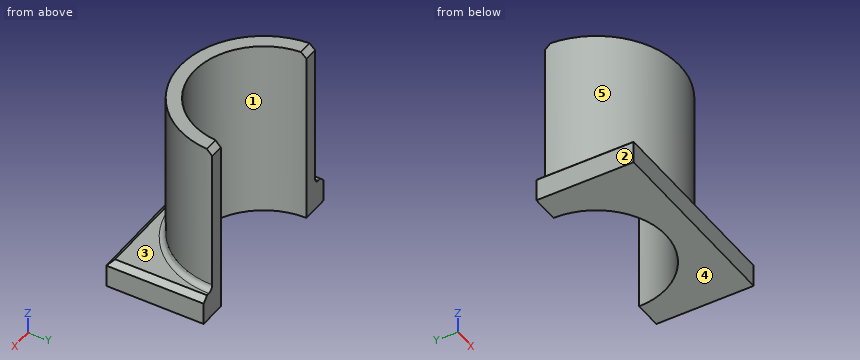
```python
from build123d import *

# Parameters (mm, degrees)
PAD_DEPTH    = 33.02
PAD001_DEPTH = 5.08
FILLET_R     = 1.016
CHAMFER_SIZE = 1


with BuildPart() as part:
    # Sketch001 → Pad (new body)
    with BuildSketch(Plane.XY):
        with BuildLine():
            ThreePointArc((-12.7, 0), (0, -12.7), (12.7, 0))
            Line((12.7, 0), (15.24, 0))
            ThreePointArc((-15.24, 0), (0, -15.24), (15.24, 0))
            Line((-15.24, 0), (-12.7, 0))
        make_face()
    extrude(amount=PAD_DEPTH)

    # Sketch → Pad001 (join)
    with BuildSketch(Plane.XY):
        with BuildLine():
            Line((-17.78, 0), (-17.78, -17.78))
            Line((-17.78, -17.78), (17.78, -17.78))
            Line((17.78, -17.78), (17.78, 0))
            Line((12.7, 0), (17.78, 0))
            ThreePointArc((-12.7, 0), (0, -12.7), (12.7, 0))
            Line((-17.78, 0), (-12.7, 0))
        make_face()
    extrude(amount=PAD001_DEPTH)

    # Fillet
    fillet_edges = [part.edges().sort_by_distance(p)[0] for p in [
        (0, -15.24, 5.08),
    ]]
    fillet(fillet_edges, radius=FILLET_R)

    # Chamfer
    chamfer_edges = [part.edges().sort_by_distance(p)[0] for p in [
        (-13.97, 0, 33.02),
        (13.97, 0, 33.02),
        (-17.78, -8.89, 5.08),
        (17.78, -8.89, 5.08),
        (0, -17.78, 5.08),
    ]]
    chamfer(chamfer_edges, length=CHAMFER_SIZE)


solid = part.part
```
Source: CAD feature listing. Evaluate the final solid. Frame: model axes, mm. Face numbers are marked on the shaded views. A direction names the side the tool comes from. Coordinates: 2 decimals unless noted, no trailing zeros. Order: outer loops, then holes, each group sorted by start corner. A loop starts at its lowest first (then second) coordinate and runs counter-clockwise, first axis right, second up. Notation, with made-up numbers: M 33,5 L 56,5 A18 ccw 56,39 Z; hole C 12,-40 d5. An arc over 180 degrees is marked long. Write each question's results on one line, items separated by ' | '. Start each with the question number.
1) Section query A-A (x = 0). Return the cut outline in (y, z).
2) Line query: line 1 (Z direction, x = -16, y = -9.25); line 2 (X direction, y = -6.75, z = 11); line 3 (X direction, y = -10.75, z = 19.5). Output: solid intervals per line, ascending. Write a range as from..to.
3) Draft query along X for the marked faces 1, 2 and 3. Return one class per face: released by +X, released by -X, zero draft, split by the parting line, or undercut.
4) Access query for the marked faces 4 and 5. Directions: +Z, -Z, +X, -X, +Y, -Y. A direction counts if a zero-diameter tool reaches every point of the face in a straight line with its end or side. Return the directions, or none.
5) Section query B-B (z = 27). Return the cut outline in (x, y), plus the area to 3 significant figures.
6) Contact query for flat-ended pins moving along their axis: pin 1 Ø3 at (y, z) = (-4.5, 8.5) entering from -X; pin 2 Ø5 at (y, z) = (-8, 13.5) entering from -X; pin 3 Ø4 at (y, z) = (-2, 21) entering from -X; pin 4 Ø8.5 at (x, y) = (-2, -10.5) entering from +Z. Output: stop coordinate, or through.
Answers:
1) outline: M -17.78,0 L -12.7,0 L -12.7,33.02 L -15.24,33.02 L -15.24,6.1 A1.02 cw -16.26,5.08 L -16.78,5.08 L -17.78,4.08 Z
2) line 1: z = 0..5.08 | line 2: x = -13.66..-10.76, 10.76..13.66 | line 3: x = -10.8..-6.76, 6.76..10.8
3) face 1: undercut | face 2: released by -X | face 3: zero draft
4) face 4: -Z, +X, -X, +Y, -Y | face 5: +Z, -Y
5) outline: M -15.24,0 A15.24 ccw 15.24,0 L 12.7,0 A12.7 cw -12.7,0 Z | area: 111 mm^2
6) pin 1: stops at x = -14.94 | pin 2: stops at x = -14.21 | pin 3: stops at x = -15.24 | pin 4: stops at z = 33.02
